Model file for the job. Use its own axes, mm. Give positions to 0.01 mm unless a question says otherwise; leave off trailing zeros. Use CSV: the item, a comma, the result in double quotes. Start each with the question number.
(1) Band-saw the part on A-A, the plane z = 1.15. Count the separate pieces of the cut face and the enclosed holes in it, then the cut area to 3 significant figures.
(2) Drop flat-ended pins along their axis: pin 1 Ø1.6 at (x, y) = (-20.77, -3.94) entering from -Z; pin 2 Ø1 at (y, z) = (-3.5, 0.5) entering from -X. Give the stop position or say it passes through.
(3) Probe L1, parallel to X at y = -3.8, z = 1.8; L2, parallel to X at y = -4.8, z = 0.3; L3, parallel to Y at x = 12.5, z = 1.85. List the from-to ranges inside material, lowest first.
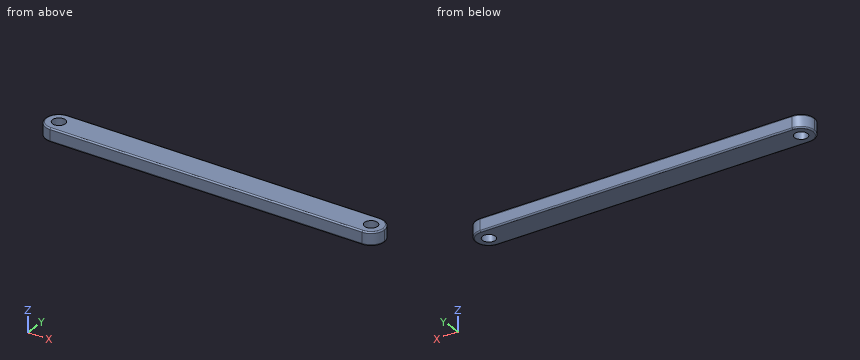
from build123d import *

# Parameters (mm, degrees)
F0_W     = 51
F0_H     = 4
F1_DEPTH = 2
F2_R     = 1.99999
F3_R     = 0.969
F4_DEPTH = 25
F5_R     = 0.2


# Not quite as in the source:
# - a fillet or chamfer is up to 0.001 mm smaller than in the source, because OpenCascade refuses the exact size


with BuildPart() as f1:
    # F0 (on Top) → F1 (new body)
    with BuildSketch(Plane.XY):
        with Locations((2.7281418443, -3.9396004599)):
            Rectangle(F0_W, F0_H)
    extrude(amount=F1_DEPTH)

    # F2 (radius 2 in the source; OpenCascade refuses exactly that, so slightly less here)
    f2_edges = [f1.edges().sort_by_distance(p)[0] for p in [
        (28.228142, -1.9396, 1),
        (28.228142, -5.9396, 1),
        (-22.771858, -1.9396, 1),
        (-22.771858, -5.9396, 1),
    ]]
    fillet(f2_edges, radius=F2_R)

    # F3 (on face) → F4 (cut)
    with BuildSketch(Plane.XY.offset(2)):
        with Locations((-20.7718581557, -3.9396004599)):
            Circle(F3_R)
        with Locations((26.2281418443, -3.9396004599)):
            Circle(F3_R)
    extrude(amount=-F4_DEPTH, mode=Mode.SUBTRACT)

    # F5
    f5_edges = [f1.edges().sort_by_distance(p)[0] for p in [
        (2.728142, -1.9396, 0),
        (2.728142, -5.9396, 2),
    ]]
    fillet(f5_edges, radius=F5_R)


solid = f1.part
Answer block:
1,separate pieces,"1"
1,enclosed holes,"2"
1,area,"195 mm2"
2,pin 1,"passes through"
2,pin 2,"stops at x = -22.77"
3,L1,"x = -22.77 to -21.73, -19.81 to 25.27, 27.19 to 28.22"
3,L2,"x = -22.58 to -21.22, -20.33 to 25.78, 26.67 to 28.03"
3,L3,"y = -5.93 to -1.95"
